from build123d import *

# Parameters (mm, degrees)
SKETCH1_W           = 76.2
SKETCH1_H           = 25.4
SKETCH1_W_2         = 69.85
SKETCH1_H_2         = 19.05
BOSS_EXTRUDE1_DEPTH = 1079.5
SKETCH2_R           = 3.3782
CUT_EXTRUDE1_DEPTH  = 26.4
SKETCH3_R           = 3.3782
CUT_EXTRUDE2_DEPTH  = 26.4
SKETCH4_R           = 3.3782
CUT_EXTRUDE3_DEPTH  = 77.2


with BuildPart() as part:
    # Sketch1 → Boss-Extrude1 (new body)
    with BuildSketch(Plane.XY):
        with Locations((38.1, 12.7)):
            Rectangle(SKETCH1_W, SKETCH1_H)
        with Locations((38.1, 12.7)):
            Rectangle(SKETCH1_W_2, SKETCH1_H_2, mode=Mode.SUBTRACT)
    extrude(amount=BOSS_EXTRUDE1_DEPTH)

    # Sketch2 → Cut-Extrude1 (cut, through all)
    with BuildSketch(Plane.XZ):
        with Locations((13.21308, 41.6687)):
            Circle(SKETCH2_R)
        with Locations((29.80436, 41.6687)):
            Circle(SKETCH2_R)
        with Locations((46.39564, 41.6687)):
            Circle(SKETCH2_R)
        with Locations((62.98692, 41.6687)):
            Circle(SKETCH2_R)
    cut_extrude1 = extrude(amount=-CUT_EXTRUDE1_DEPTH, mode=Mode.SUBTRACT)

    # Mirror1: Cut-Extrude1 across plane
    add(cut_extrude1.mirror(Plane(origin=(0, 0, 539.75), x_dir=(1, 0, 0), z_dir=(0, 0, -1))), mode=Mode.SUBTRACT)

    # Sketch3 → Cut-Extrude2 (cut, through all)
    with BuildSketch(Plane(origin=(0, 25.4, 0), x_dir=(1, 0, 0), z_dir=(0, 1, 0))):
        with Locations((13.21308, -789.3812)):
            Circle(SKETCH3_R)
        with Locations((29.80436, -789.3812)):
            Circle(SKETCH3_R)
        with Locations((46.39564, -789.3812)):
            Circle(SKETCH3_R)
        with Locations((62.98692, -789.3812)):
            Circle(SKETCH3_R)
        with Locations((29.80436, -680.6438)):
            Circle(SKETCH3_R)
        with Locations((46.39564, -680.6438)):
            Circle(SKETCH3_R)
        with Locations((62.98692, -680.6438)):
            Circle(SKETCH3_R)
        with Locations((13.21308, -290.1188)):
            Circle(SKETCH3_R)
        with Locations((29.80436, -290.1188)):
            Circle(SKETCH3_R)
        with Locations((46.39564, -290.1188)):
            Circle(SKETCH3_R)
        with Locations((62.98692, -290.1188)):
            Circle(SKETCH3_R)
        with Locations((13.21308, -398.8562)):
            Circle(SKETCH3_R)
        with Locations((29.80436, -398.8562)):
            Circle(SKETCH3_R)
        with Locations((46.39564, -398.8562)):
            Circle(SKETCH3_R)
        with Locations((62.98692, -398.8562)):
            Circle(SKETCH3_R)
        with Locations((13.21308, -680.6438)):
            Circle(SKETCH3_R)
    extrude(amount=-CUT_EXTRUDE2_DEPTH, mode=Mode.SUBTRACT)

    # Sketch4 → Cut-Extrude3 (cut, through all)
    with BuildSketch(Plane.ZY):
        with Locations((710.12558, 9.1313)):
            Circle(SKETCH4_R)
        with Locations((759.89942, 9.1313)):
            Circle(SKETCH4_R)
        with Locations((743.30814, 9.1313)):
            Circle(SKETCH4_R)
        with Locations((726.71686, 9.1313)):
            Circle(SKETCH4_R)
    cut_extrude3 = extrude(amount=-CUT_EXTRUDE3_DEPTH, mode=Mode.SUBTRACT)

    # Mirror2: Cut-Extrude3 across plane
    add(cut_extrude3.mirror(Plane(origin=(0, 0, 539.75), x_dir=(1, 0, 0), z_dir=(0, 0, -1))), mode=Mode.SUBTRACT)


solid = part.part
Source: CAD feature listing. Evaluate the final solid. Frame: model axes, mm. A direction names the side the tool comes from. Coordinates: 2 decimals unless noted, no trailing zeros. Write each loop counter-clockwise with the first axis right and the second up, starting at its lowest first coordinate (ties: lowest second). Pieces come first, ordered by that corner, then holes. Notation, with made-up numbers: M 18.25,78 L 70.25,78 A10 ccw 70.25,85 Z; hole C 65.5,88 d11. An arc over 180 degrees is marked long. Use a Markdown table: item, result.
1) First-contact query: pin 1 Ø12 at (x, y) = (54, 7.5) entering from +Z; pin 2 Ø6 at (x, z) = (13.21, 1037.83) entering from +Y. Flat tips, straight axial feed; report the tip coordinate or a pass-through.
Conclusion:
| item | result |
|---|---|
| pin 1 | stops at z = 1079.5 |
| pin 2 | passes through |
2) Ray query, L1, parallel to Y at x = 5, z = 169 (3 decimals); L2, parallel to X at y = 4.25, z = 120 (3 decimals). Return the intervals inside material, ascending.
Conclusion:
| item | result |
|---|---|
| L1 | y = 0 to 3.175, 22.225 to 25.4 |
| L2 | x = 0 to 3.175, 73.025 to 76.2 |
3) Reachability of faces 4 (the flat face through (76.2, 13, 532)), 5 (the flat face through (38, 22.225, 532)) from +Z, -Z, +X, -X, +Y, -Y: full face, straight path, thin tool, end or side. Return the list, or none.
Conclusion:
| item | result |
|---|---|
| face 4 | +Z, -Z, +X, +Y, -Y |
| face 5 | +Z, -Z |
4) Section A-A, the plane y = 17.5. Output: boundary loops of the cut face in (x, z) (3 decimals), then the cut area to 3 significant figures.
Conclusion:
| item | result |
|---|---|
| outline | M 0,0 L 3.175,0 L 3.175,1079.5 L 0,1079.5 Z; M 73.025,0 L 76.2,0 L 76.2,1079.5 L 73.025,1079.5 Z |
| area | 6,850 mm^2 |
5) Mould query, pull axis Y, two halves, no side actions, for faces 1 (the flat face through (35, 2, 1079.5)), 2 (the flat face through (38, 25.4, 532)), 3 (the flat face through (38, 3.175, 532)). Classes: pulls with the +Y half, pulls with the -Y half, needs draft (parallel to the pull), parting line crosses it, or undercut.
Conclusion:
| item | result |
|---|---|
| face 1 | needs draft |
| face 2 | pulls with the +Y half |
| face 3 | undercut |
6) Section B-B, the plane z = 196.5. Output: boundary loops of the cut face in (x, y) (3 decimals), then the cut area to 3 significant figures.
Conclusion:
| item | result |
|---|---|
| outline | M 0,0 L 76.2,0 L 76.2,25.4 L 0,25.4 Z; hole M 3.175,3.175 L 73.025,3.175 L 73.025,22.225 L 3.175,22.225 Z |
| area | 605 mm^2 |
